from build123d import *

# Parameters (mm, degrees)
F0_W          = 6.714124
F0_H          = 36.647938
F1_DEPTH      = 69.85
F1_DEPTH_BACK = 66.294
F2_R          = 17.783097
F3_R          = 17.78
F4_R          = 17.78


with BuildPart() as f1:
    # F0 (on Front) → F1 (new body, two sides)
    with BuildSketch(Plane.XZ) as f1_sk:
        Rectangle(F0_W, F0_H)
    extrude(amount=F1_DEPTH)
    extrude(f1_sk.sketch, amount=-F1_DEPTH_BACK)

    # F2
    f2_edges = [f1.edges().sort_by_distance(p)[0] for p in [
        (0, -69.85, 18.323969),
    ]]
    fillet(f2_edges, radius=F2_R)

    # F3
    f3_edges = [f1.edges().sort_by_distance(p)[0] for p in [
        (0, -69.85, -18.323969),
    ]]
    fillet(f3_edges, radius=F3_R)

    # F4
    f4_edges = [f1.edges().sort_by_distance(p)[0] for p in [
        (0, 66.294, -18.323969),
        (0, 66.294, 18.323969),
    ]]
    fillet(f4_edges, radius=F4_R)


solid = f1.part
Verification items for the finished model (mm, model axes). Give positions to 0.01 mm unless a question says otherwise; leave off trailing zeros. Write each loop counter-clockwise with the first axis right and the second up, starting at its lowest first coordinate (ties: lowest second). Pieces come first, ordered by that corner, then holes.
(1) Cross-section at B-B (z = 16). Enter the section's corners in (x, y), plus the area to 3 significant figures.
(2) Material ranges on line 1 (Y direction, x = 1.5, z = 1.5); line 2 (Y direction, x = 0.5, z = -2); line 3 (Z direction, x = -2.25, y = -57), recorded low to high.
(3) Cross-section at A-A (x = -1.75). Enter the section's corners in (y, z).
(4) Cross-section at C-C (y = 52). Enter the section's corners in (x, z), plus the area to 3 significant figures.
(5) Gauge pin test, flat ends, axial feed: pin 1 (2 mm diameter, centred on x = -1.5, z = -14, fed in from -Y); pin 2 (1 mm diameter, centred on x = -0.5, z = 10.5, fed in from -Y). Record the tip position at first contact, or that the pin passes through.
Worked out:
1. outline: (-3.36, -60.86) - (3.36, -60.86) - (3.36, 57.3) - (-3.36, 57.3) - close
1. area: 793 mm2
2. line 1: y = -69.82 to 66.27
2. line 2: y = -69.79 to 66.23
2. line 3: z = -17.63 to 17.63
3. outline: (-69.85, -0.54) arc R17.78 ccw to (-52.07, -18.32) - (48.51, -18.32) arc R17.78 ccw to (66.29, -0.54) - (66.29, 0.54) arc R17.78 ccw to (48.51, 18.32) - (-52.07, 18.32) arc R17.78 ccw to (-69.85, 0.54) - close
4. outline: (-3.36, -17.98) - (3.36, -17.98) - (3.36, 17.98) - (-3.36, 17.98) - close
4. area: 241 mm2
5. pin 1: stops at y = -64.76
5. pin 2: stops at y = -67.13
